The listing builds one solid part. Answer for the finished solid, in the listing's coordinates (mm). Give positions to 0.01 mm unless a question says otherwise; leave off trailing zeros. Order: outer loops, then holes, each group sorted by start corner. A loop starts at its lowest first (then second) coordinate and runs counter-clockwise, first axis right, second up. Notation, with made-up numbers: (24, 7.5) - (47, 7.5) arc R17 ccw to (47, 36.5) - close; hole circle Ø6 at (-20, 37.5). An arc over 180 degrees is marked (long way). Answer in a Markdown table with one row per item. Add a question column.
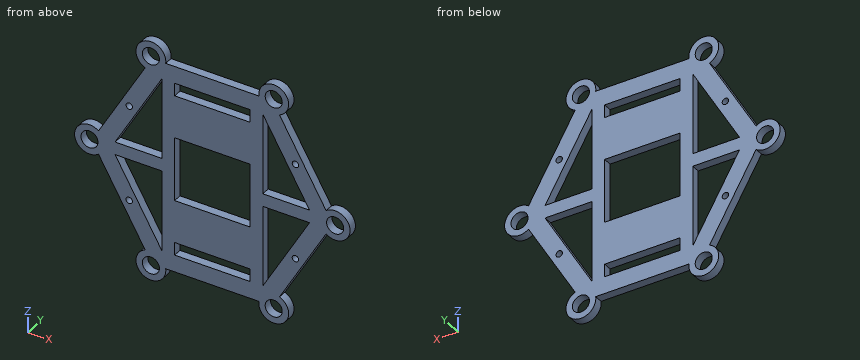
```python
from build123d import *

# Parameters (mm, degrees)
SKETCH_1_R          = 4
SKETCH_1_R_2        = 1.5
SKETCH_1_W          = 35.342722074
SKETCH_1_H          = 6
SKETCH_1_H_2        = 30
EXTRUDE_1_DEPTH     = 4
CUT_EXTRUDE_START   = -2
SKETCH_2_R          = 7
CUT_EXTRUDE_1_DEPTH = 1.1


with BuildPart() as part:
    # 草图1 → 凸台-拉伸1 (new body)
    with BuildSketch(Plane(origin=(0, 0, 0), x_dir=(1, 0, 0), z_dir=(0, 1, 0))):
        with BuildLine():
            ThreePointArc((-21.862962012, 49), (-32.305762114, 55.955221358), (-31.503763779, 43.433880504))
            Line((-31.503763779, 43.433880504), (-53.366725791, 5.566119496))
            ThreePointArc((-53.366725791, 5.566119496), (-64.611524227, 0), (-53.366725791, -5.566119496))
            Line((-53.366725791, -5.566119496), (-31.503763779, -43.433880504))
            ThreePointArc((-31.503763779, -43.433880504), (-32.305762114, -55.955221358), (-21.862962012, -49))
            Line((-21.862962012, -49), (21.862962012, -49))
            ThreePointArc((21.862962012, -49), (32.305762114, -55.955221358), (31.503763779, -43.433880504))
            Line((31.503763779, -43.433880504), (53.366725791, -5.566119496))
            ThreePointArc((53.366725791, -5.566119496), (64.611524227, 0), (53.366725791, 5.566119496))
            Line((53.366725791, 5.566119496), (31.503763779, 43.433880504))
            ThreePointArc((31.503763779, 43.433880504), (32.305762114, 55.955221358), (21.862962012, 49))
            Line((21.862962012, 49), (-21.862962012, 49))
        make_face()
        with Locations((-28.805762114, 49.893043531)):
            Circle(SKETCH_1_R, mode=Mode.SUBTRACT)
        with Locations((28.805762114, -49.893043531)):
            Circle(SKETCH_1_R, mode=Mode.SUBTRACT)
        with Locations((-28.805762114, -49.893043531)):
            Circle(SKETCH_1_R, mode=Mode.SUBTRACT)
        with Locations((-57.611524227, 0)):
            Circle(SKETCH_1_R, mode=Mode.SUBTRACT)
        with Locations((38.97114317, 22.5)):
            Circle(SKETCH_1_R_2, mode=Mode.SUBTRACT)
        with Locations((-38.97114317, -22.5)):
            Circle(SKETCH_1_R_2, mode=Mode.SUBTRACT)
        with Locations((0, 38)):
            Rectangle(SKETCH_1_W, SKETCH_1_H, mode=Mode.SUBTRACT)
        Rectangle(SKETCH_1_W, SKETCH_1_H_2, mode=Mode.SUBTRACT)
        with Locations((0, -38)):
            Rectangle(SKETCH_1_W, SKETCH_1_H, mode=Mode.SUBTRACT)
        Polygon((23.671361037, 41), (45.610671266, 3), (23.671361037, 3), align=None, mode=Mode.SUBTRACT)
        Polygon((45.610671266, -3), (23.671361037, -41), (23.671361037, -3), align=None, mode=Mode.SUBTRACT)
        Polygon((-23.671361037, -41), (-45.610671266, -3), (-23.671361037, -3), align=None, mode=Mode.SUBTRACT)
        Polygon((-45.610671266, 3), (-23.671361037, 41), (-23.671361037, 3), align=None, mode=Mode.SUBTRACT)
        with Locations((38.97114317, -22.5)):
            Circle(SKETCH_1_R_2, mode=Mode.SUBTRACT)
        with Locations((-38.97114317, 22.5)):
            Circle(SKETCH_1_R_2, mode=Mode.SUBTRACT)
        with Locations((28.805762114, 49.893043531)):
            Circle(SKETCH_1_R, mode=Mode.SUBTRACT)
        with Locations((57.611524227, 0)):
            Circle(SKETCH_1_R, mode=Mode.SUBTRACT)
    extrude(amount=EXTRUDE_1_DEPTH)

    # 草图2 → 切除-拉伸1 (cut)
    with BuildSketch(Plane(origin=(0, 4, 0), x_dir=(1, 0, 0), z_dir=(0, 1, 0)).offset(CUT_EXTRUDE_START)):
        with Locations((0, 25)):
            Circle(SKETCH_2_R)
        with Locations((-0.013100305, -25.004400745)):
            Circle(SKETCH_2_R)
    extrude(amount=CUT_EXTRUDE_1_DEPTH, mode=Mode.SUBTRACT)


solid = part.part
```
(1) Find section C-C, the plane z = 0. Write down the section's boundary in (x, y), plus the area to 3 significant figures.
(2) Each of these flat-tipped pins is pushed along its axis until it touches: P1, Ø2, axis at x = 33.5, y = 0.5, coming from the +Z side; P2, Ø10, axis at x = -3, z = 37.5, coming from the +Y side; P3, Ø1.2, axis at x = 32.5, y = 3, coming from the +Z side; P4, Ø2, axis at y = 2.5, z = 26, coming from the -X side. Where does it stop, or does it pass through?
(3) Find section A-A, the plane x = -5.5. Write down the section's boundary in (y, z), plus the area to 3 significant figures.
(4) Find section D-D, the plane x = 48. Write down the section's boundary in (y, z), plus the area to 3 significant figures.
(5) Find section B-B, the plane z = -37. Write down the section's boundary in (x, y), plus the area to 3 significant figures.
(6) Straight lines are drawn through the part: line 1 (Z direction, x = -6, y = 1.3); line 2 (Z direction, x = 24, y = 1.5); line 3 (Z direction, x = -25.5, y = 3.1). For each, find the intervals that lie inside material, in ascending order.
Answer key:
| question | item | result |
|---|---|---|
| 1 | outline | (-64.61, 0) - (-61.61, 0) - (-61.61, 4) - (-64.61, 4) - close; (-53.61, 0) - (-17.67, 0) - (-17.67, 4) - (-53.61, 4) - close; (17.67, 0) - (53.61, 0) - (53.61, 4) - (17.67, 4) - close; (61.61, 0) - (64.61, 0) - (64.61, 4) - (61.61, 4) - close |
| 1 | area | 312 mm² |
| 2 | P1 | z = 55.84 |
| 2 | P2 | y = 4 |
| 2 | P3 | z = 56.17 |
| 2 | P4 | x = -42.15 |
| 3 | outline | (0, -49) - (4, -49) - (4, -41) - (0, -41) - close; (0, -35) - (4, -35) - (4, -15) - (0, -15) - close; (0, 15) - (4, 15) - (4, 35) - (0, 35) - close; (0, 41) - (4, 41) - (4, 49) - (0, 49) - close; hole (2, -29.33) - (3.1, -29.33) - (3.1, -20.67) - (2, -20.67) - close; hole (2, 20.66) - (3.1, 20.66) - (3.1, 29.35) - (2, 29.35) - close |
| 3 | area | 205 mm² |
| 4 | outline | (0, -14.86) - (4, -14.86) - (4, 14.86) - (0, 14.86) - close |
| 4 | area | 119 mm² |
| 5 | outline | (-35.22, 0) - (-25.98, 0) - (-25.98, 4) - (-35.22, 4) - close; (-23.67, 0) - (-17.67, 0) - (-17.67, 4) - (-23.67, 4) - close; (17.67, 0) - (23.67, 0) - (23.67, 4) - (17.67, 4) - close; (25.98, 0) - (35.22, 0) - (35.22, 4) - (25.98, 4) - close |
| 5 | area | 122 mm² |
| 6 | line 1 | -49 to -41, -35 to -15, 15 to 35, 41 to 49 |
| 6 | line 2 | -54.98 to -40.43, -3 to 3, 40.43 to 54.98 |
| 6 | line 3 | -56.06 to -52.15, -47.64 to -37.83, -3 to 3, 37.83 to 47.64, 52.15 to 56.06 |
